from build123d import *

# Parameters (mm, degrees)
SKETCH1_W                                      = 60.6552
SKETCH1_H                                      = 128.4986
BOSS_EXTRUDE1_DEPTH                            = 2.54
CSK_FOR_M3_FLAT_HEAD_MACHINE_SCREW1_AT_2_COUNT = 2
CSK_FOR_M3_FLAT_HEAD_MACHINE_SCREW1_AT_2_PITCH = 75.0062
M2_5_CLEARANCE_SLOT1_DEPTH                     = 2.54
F_1_4_CLEARANCE_HOLE1_D                        = 7.14248
F_1_4_CLEARANCE_HOLE2_D                        = 6.5278
F_3_8_CLEARANCE_HOLE2_D                        = 10.0838
F_10_CLEARANCE_HOLE1_D                         = 5.6134


# Read off the part's stored shape, not the designer's step: M2.5 Clearance Slot1
with BuildPart() as part:
    # Sketch1 → Boss-Extrude1 (new body)
    with BuildSketch(Plane(origin=(0, 0, 0), x_dir=(1, 0, 0), z_dir=(0, 1, 0))):
        Rectangle(SKETCH1_W, SKETCH1_H)
    extrude(amount=BOSS_EXTRUDE1_DEPTH)

    # Sketch5 → CSK for M3 Flat Head Machine Screw1 (revolve, cut)
    with BuildSketch(Plane(origin=(25.4, 0, -37.5031), x_dir=(0, 0, -1), z_dir=(1, 0, 0))):
        Polygon((0, 0), (0, 2.54), (1.8, 2.54), (1.8, 1.35), (3.15, 0), align=None)
    csk_for_m3_flat_head_machine_screw1 = revolve(axis=Axis((25.4, -6.35, -37.5031), (0, 1, 0)), mode=Mode.SUBTRACT)

    # CSK for M3 Flat Head Machine Screw1 at 2: CSK for M3 Flat Head Machine Screw1 ×2
    with Locations(*[(0, 0, i * CSK_FOR_M3_FLAT_HEAD_MACHINE_SCREW1_AT_2_PITCH) for i in range(1, CSK_FOR_M3_FLAT_HEAD_MACHINE_SCREW1_AT_2_COUNT)]):
        add(csk_for_m3_flat_head_machine_screw1, mode=Mode.SUBTRACT)

    # M2.5 Clearance Slot1 outline → M2.5 Clearance Slot1 (cut)
    with BuildSketch(Plane(origin=(0, 0, 0), x_dir=(1, 0, 0), z_dir=(0, 1, 0))):
        with BuildLine():
            ThreePointArc((23.36, -62.7021), (24.81, -61.2521), (23.36, -59.8021))
            Line((23.36, -59.8021), (22.36, -59.8021))
            ThreePointArc((22.36, -59.8021), (20.91, -61.2521), (22.36, -62.7021))
            Line((22.36, -62.7021), (23.36, -62.7021))
        make_face()
        with BuildLine():
            ThreePointArc((23.36, 59.8021), (24.81, 61.2521), (23.36, 62.7021))
            Line((23.36, 62.7021), (22.36, 62.7021))
            ThreePointArc((22.36, 62.7021), (20.91, 61.2521), (22.36, 59.8021))
            Line((22.36, 59.8021), (23.36, 59.8021))
        make_face()
    m2_5_clearance_slot1 = extrude(amount=M2_5_CLEARANCE_SLOT1_DEPTH, mode=Mode.SUBTRACT)

    # Mirror1: CSK for M3 Flat Head Machine Screw1, M2.5 Clearance Slot1 across plane
    add(csk_for_m3_flat_head_machine_screw1.mirror(Plane(origin=(0, 0, 0), x_dir=(0, 0, 1), z_dir=(1, 0, 0))), mode=Mode.SUBTRACT)
    add(m2_5_clearance_slot1.mirror(Plane(origin=(0, 0, 0), x_dir=(0, 0, 1), z_dir=(1, 0, 0))), mode=Mode.SUBTRACT)

    # Mirror1 copy 1 sketch → Mirror1 copy 1 (revolve, cut)
    with BuildSketch(Plane(origin=(-25.4, 0, 37.5031), x_dir=(0, 0, -1), z_dir=(-1, 0, 0))):
        Polygon((0, 0), (0, -2.54), (1.8, -2.54), (1.8, -1.35), (3.15, 0), align=None)
    revolve(axis=Axis((-25.4, -6.35, 37.5031), (0, -1, 0)), mode=Mode.SUBTRACT)

    # 1/4 Clearance Hole1 (through all)
    with Locations(Plane(origin=(0, 0, 0), x_dir=(-1, 0, 0), z_dir=(0, -1, 0))):
        with Locations((18.6436, 35.0012), (18.6436, 21.301199968), (18.6436, -35.0012)):
            Hole(F_1_4_CLEARANCE_HOLE1_D / 2)

    # 1/4 Clearance Hole2 (through all)
    with Locations(Plane(origin=(0, 0, 0), x_dir=(-1, 0, 0), z_dir=(0, -1, 0))):
        with Locations((-18.4404, 35.0012), (5.9436, 35.0012), (5.9436, 21.301199968), (-18.4404, 21.301199968), (-18.6436, -17.091200006), (0, -35.0012)):
            Hole(F_1_4_CLEARANCE_HOLE2_D / 2)

    # 3/8 Clearance Hole2 (through all)
    with Locations(Plane(origin=(0, 0, 0), x_dir=(-1, 0, 0), z_dir=(0, -1, 0))):
        with Locations((12.0396, -17.091200006), (-6.2484, 2.731200024)):
            Hole(F_3_8_CLEARANCE_HOLE2_D / 2)

    # #10 Clearance Hole1 (through all)
    with Locations(Plane(origin=(0, 0, 0), x_dir=(-1, 0, 0), z_dir=(0, -1, 0))):
        with Locations((14.224, -4.268799946), (14.224, 2.731200024), (14.224, 9.731199994), (-18.6436, -35.0012)):
            Hole(F_10_CLEARANCE_HOLE1_D / 2)


solid = part.part
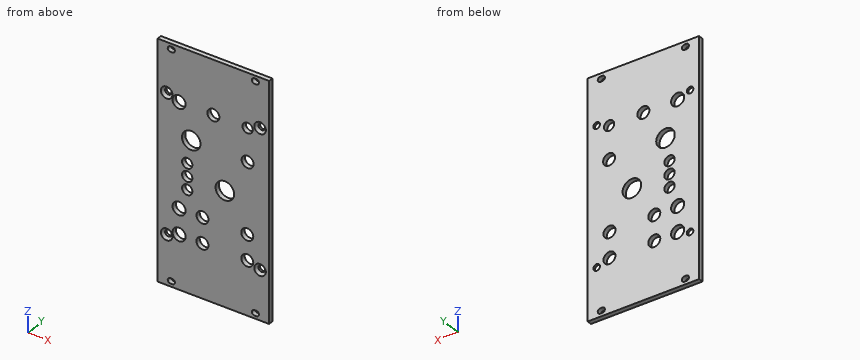
The listing builds one solid part. Answer for the finished solid, in the listing's coordinates (mm). Coordinates: 2 decimals unless noted, no trailing zeros. Write each loop counter-clockwise with the first axis right and the second up, starting at its lowest first coordinate (ties: lowest second). Pieces come first, ordered by that corner, then holes. Notation, with made-up numbers: (24.5, 63.5) - (82.5, 63.5) arc R20 cw to (82.5, 82.5) - close; hole circle Ø6 at (-17.75, -6.75). An arc over 180 degrees is marked (long way). Answer as CSV lines item,"result".
1. Straight lines are drawn through the part: line 1 (Z direction, x = 22, y = 2); line 2 (X direction, y = 0.8, z = 35); line 3 (Z direction, x = 2, y = 0.65). For each, find the intervals that lie inside material, in ascending order. Write a range as [from, to].
Computed values:
line 1,"z = [-64.25, -62.66], [-59.85, 59.85], [62.66, 64.25]"
line 2,"x = [-30.33, -22.21], [-15.07, -3.26], [3.26, 15.84], [21.45, 30.33]"
line 3,"z = [-64.25, -5.45], [-0.02, 32.42], [37.58, 64.25]"
2. Given P1, Ø4, axis at x = -25.4, z = -37.5, coming from the -Y side, flat-ended and moving along its own axis, determine where the tip first touches the part or whether it passes through.
Computed values:
P1,"stops at y = 1.15"
3. Find section B-B (y = 0.6). Give the number of separate pieces and of enclosed holes in the cut face, plus the area to 3 significant figures.
Computed values:
separate pieces,"1"
enclosed holes,"23"
area,"7,090 mm²"
4. Find section A-A (x = 0). Give the vertices of the cut face in (y, z).
Computed values:
outline,"(0, -64.25) - (2.54, -64.25) - (2.54, 31.74) - (0, 31.74) - close; (0, 38.27) - (2.54, 38.27) - (2.54, 64.25) - (0, 64.25) - close"
